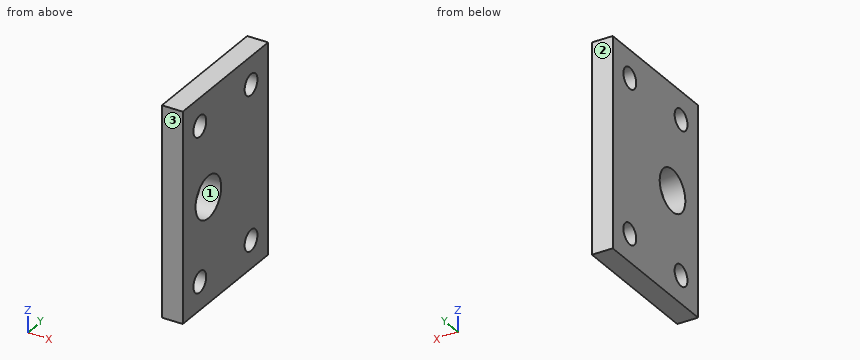
```python
from build123d import *

# Parameters (mm, degrees)
SKETCH_1_W          = 30
SKETCH_1_H          = 20
SKETCH_1_R          = 1.5
EXTRUDE_1_DEPTH     = 3
CUT_EXTRUDE_1_REACH = 5
SKETCH_2_R          = 3


with BuildPart() as part:
    # 草图1 → 凸台-拉伸1 (new body)
    with BuildSketch(Plane(origin=(0, 0, 0), x_dir=(0, 0, -1), z_dir=(1, 0, 0))):
        Rectangle(SKETCH_1_W, SKETCH_1_H)
        with Locations((-11, 6)):
            Circle(SKETCH_1_R, mode=Mode.SUBTRACT)
        with Locations((-11, -6)):
            Circle(SKETCH_1_R, mode=Mode.SUBTRACT)
        with Locations((11, -6)):
            Circle(SKETCH_1_R, mode=Mode.SUBTRACT)
        with Locations((11, 6)):
            Circle(SKETCH_1_R, mode=Mode.SUBTRACT)
    extrude(amount=EXTRUDE_1_DEPTH)

    # 草图2 → 切除-拉伸1 (cut, up to next)
    with BuildSketch(Plane.ZY, mode=Mode.PRIVATE) as cut_extrude_1_sk1:
        with Locations((0, -4)):
            Circle(SKETCH_2_R)
    cut_extrude_1_tool1 = extrude(cut_extrude_1_sk1.sketch, amount=-CUT_EXTRUDE_1_REACH, mode=Mode.PRIVATE) & part.part
    add(cut_extrude_1_tool1.solids().sort_by_distance((0, -4, 0))[0], mode=Mode.SUBTRACT)


solid = part.part
```
Input: part model. Units: mm. Frame: model coordinates. Face numbers are marked on the shaded views. Give positions to 0.01 mm unless a question says otherwise; leave off trailing zeros. Loops run counter-clockwise (first coordinate to the right, second up) from the corner with the lowest first, then second, coordinate; pieces in that order, holes last.
1) Section query A-A on z = -11. Return the cut outline in (x, y), and give its area (3 significant figures).
A:
outline: (0, -10) - (3, -10) - (3, -7.5) - (0, -7.5) - close; (0, -4.5) - (3, -4.5) - (3, 4.5) - (0, 4.5) - close; (0, 7.5) - (3, 7.5) - (3, 10) - (0, 10) - close
area: 42.0 mm2
2) Contact query for a flat-ended pin moving along its axis: pin 1 (1.8 mm diameter, centred on y = -6, z = -11, fed in from -X). Output: stop coordinate, or through.
A:
pin 1: passes through
3) Section query B-B on x = 2.1. Return the cut outline in (y, z).
A:
outline: (-10, -15) - (10, -15) - (10, 15) - (-10, 15) - close; hole circle Ø3 at (-6, -11); hole circle Ø3 at (-6, 11); hole circle Ø6 at (-4, 0); hole circle Ø3 at (6, -11); hole circle Ø3 at (6, 11)
4) Line query: L1, parallel to Y at x = 1.65, z = 11; L2, parallel to Y at x = 1.5, z = 0; L3, parallel to Z at x = 0.55, y = -4.75. Output: solid intervals per line, ascending.
A:
L1: y = -10 to -7.5, -4.5 to 4.5, 7.5 to 10
L2: y = -10 to -7, -1 to 10
L3: z = -15 to -11.83, -10.17 to -2.9, 2.9 to 10.17, 11.83 to 15
5) Mould query, pull axis Y, two halves, no side actions, for the marked faces 1, 2 and 3. Classes: released by +Y, released by -Y, zero draft, split by the parting line, or undercut.
A:
face 1: undercut
face 2: released by +Y
face 3: released by -Y
6) Section query C-C on y = -4. Return the cut outline in (x, z).
A:
outline: (0, -15) - (3, -15) - (3, -3) - (0, -3) - close; (0, 3) - (3, 3) - (3, 15) - (0, 15) - close
7) Section query D-D on z = 0. Return the cut outline in (x, y).
A:
outline: (0, -10) - (3, -10) - (3, -7) - (0, -7) - close; (0, -1) - (3, -1) - (3, 10) - (0, 10) - close
